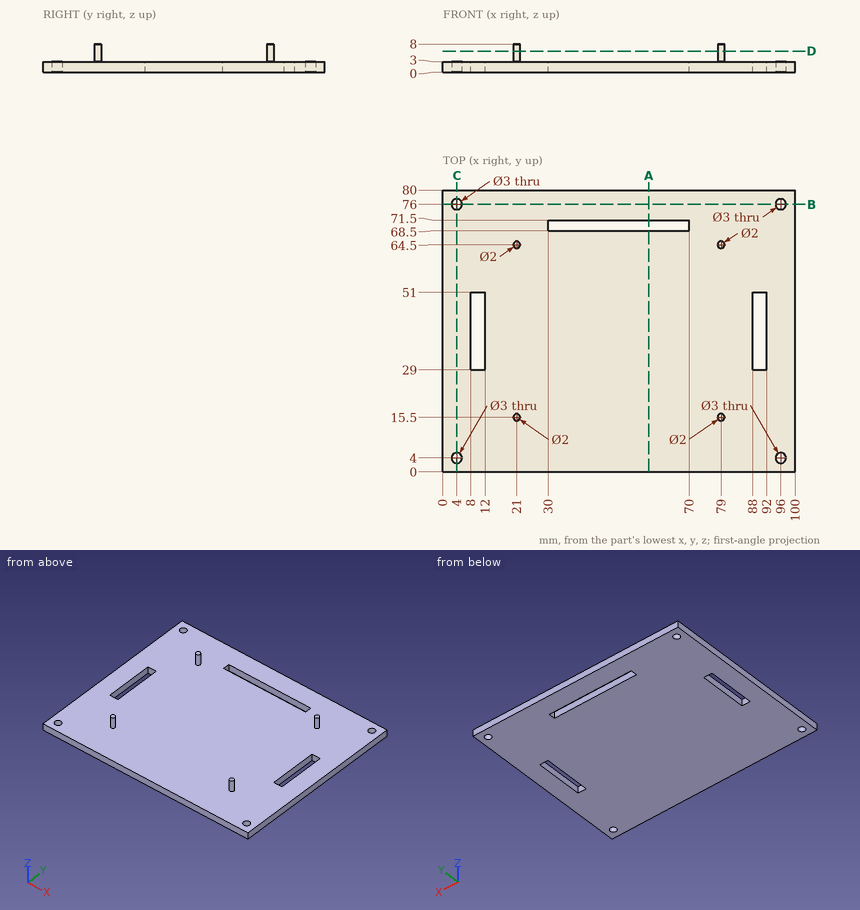
Source: three-view drawing plus pictorial views. Frame: mm from the lowest corner of the part. Coordinates: 2 decimals unless noted, no trailing zeros. Order: outer loops, then holes, each group sorted by start corner. A loop starts at its lowest first (then second) coordinate and runs counter-clockwise, first axis right, second up.
Item 1: Cut plane D-D (z = 6). Return loops of the section in (x, y), plus the area to 3 significant figures.
Output values:
outline: circle Ø2 at (21, 15.5); circle Ø2 at (21, 64.5); circle Ø2 at (79, 15.5); circle Ø2 at (79, 64.5)
area: 12.6 mm2
Item 2: Cut plane B-B (y = 76). Return loops of the section in (x, z).
Output values:
outline: (0, 0) - (2.5, 0) - (2.5, 3) - (0, 3) - close; (5.5, 0) - (94.5, 0) - (94.5, 3) - (5.5, 3) - close; (97.5, 0) - (100, 0) - (100, 3) - (97.5, 3) - close
Item 3: First-contact query: P1, Ø12, axis at x = 38, y = 29.5, coming from the +Z side; P2, Ø1.8, axis at x = 4, y = 4, coming from the +Z side. Flat tips, straight axial feed; report the tip coordinate or a pass-through.
Output values:
P1: stops at z = 3
P2: passes through
Item 4: Cut plane A-A (x = 58.5). Return loops of the section in (y, z), plus the area to 3 significant figures.
Output values:
outline: (0, 0) - (68.5, 0) - (68.5, 3) - (0, 3) - close; (71.5, 0) - (80, 0) - (80, 3) - (71.5, 3) - close
area: 231 mm2
Item 5: Material intervals for line 1 (Y direction, x = 4, z = 1.75); line 2 (X direction, y = 76, z = 0.75); line 3 (X direction, y = 49, z = 2.75), sorted ascending.
Output values:
line 1: y = 0 to 2.5, 5.5 to 74.5, 77.5 to 80
line 2: x = 0 to 2.5, 5.5 to 94.5, 97.5 to 100
line 3: x = 0 to 8, 12 to 88, 92 to 100
Item 6: Cut plane C-C (x = 4). Return loops of the section in (y, z), plus the area to 3 significant figures.
Output values:
outline: (0, 0) - (2.5, 0) - (2.5, 3) - (0, 3) - close; (5.5, 0) - (74.5, 0) - (74.5, 3) - (5.5, 3) - close; (77.5, 0) - (80, 0) - (80, 3) - (77.5, 3) - close
area: 222 mm2
